Build history of the part. All positions in model axes, mm. Face numbers are marked on the shaded views. A direction names the side the tool comes from. Round coordinates to 2 decimals unless told otherwise and drop trailing zeros. Write each loop counter-clockwise with the first axis right and the second up, starting at its lowest first coordinate (ties: lowest second). Pieces come first, ordered by that corner, then holes. Notation, with made-up numbers: M 41,37.25 L 80,37.25 A16 cw 80,51.25 Z; hole C -13.75,66 d2. An arc over 180 degrees is marked long. Write item = value, one per line.
from build123d import *

# Parameters (mm, degrees)
SKETCH2_W                 = 39
SKETCH2_H                 = 29
BOSS_EXTRUDE1_DEPTH       = 14.5
SKETCH4_R                 = 14
BOSS_EXTRUDE2_DEPTH       = 6.5
SKETCH5_R                 = 21
BOSS_EXTRUDE3_DEPTH       = 40
SKETCH6_R                 = 27
BOSS_EXTRUDE4_DEPTH       = 15.5
M3X0_5_TAPPED_HOLE1_D     = 2.5
M3X0_5_TAPPED_HOLE1_DEPTH = 5
M3X0_5_TAPPED_HOLE1_TIP   = 0.751075774


with BuildPart() as part:
    # Sketch2 → Boss-Extrude1 (new, symmetric)
    with BuildSketch(Plane(origin=(0, 0, 0), x_dir=(1, 0, 0), z_dir=(0, 1, 0))):
        Rectangle(SKETCH2_W, SKETCH2_H)
    extrude(amount=BOSS_EXTRUDE1_DEPTH, both=True)

    # Sketch4 → Boss-Extrude2 (add)
    with BuildSketch(Plane(origin=(19.5, 0, 0), x_dir=(0, 0, -1), z_dir=(1, 0, 0))):
        with Locations(Location((0, 0, 0), (0, 0, 180))):
            Circle(SKETCH4_R)
    extrude(amount=BOSS_EXTRUDE2_DEPTH)

    # Sketch5 → Boss-Extrude3 (add)
    with BuildSketch(Plane(origin=(26, 0, 0), x_dir=(0, 0, -1), z_dir=(1, 0, 0))):
        Circle(SKETCH5_R)
    extrude(amount=BOSS_EXTRUDE3_DEPTH)

    # Sketch6 → Boss-Extrude4 (add)
    with BuildSketch(Plane(origin=(66, 0, 0), x_dir=(0, 0, -1), z_dir=(1, 0, 0))):
        Circle(SKETCH6_R)
    extrude(amount=BOSS_EXTRUDE4_DEPTH)

    # M3x0.5 Tapped Hole1
    with Locations(Plane(origin=(0, -14.5, 0), x_dir=(-1, 0, 0), z_dir=(0, -1, 0))):
        with Locations((-16.5, 11.5), (16.5, 11.5), (16.5, -11.5), (-16.5, -11.5)):
            Hole(M3X0_5_TAPPED_HOLE1_D / 2, depth=M3X0_5_TAPPED_HOLE1_DEPTH)
            with Locations((0, 0, -(M3X0_5_TAPPED_HOLE1_DEPTH + M3X0_5_TAPPED_HOLE1_TIP / 2))):  # 118° drill point
                Cone(0, M3X0_5_TAPPED_HOLE1_D / 2, M3X0_5_TAPPED_HOLE1_TIP, mode=Mode.SUBTRACT)

    # Sketch12 → Revolve1 (revolve)
    with BuildSketch(Plane.XY, mode=Mode.PRIVATE) as revolve1_sk:
        Polygon((61.5, 0), (141.5, 67.127970494), (141.5, 0), align=None)
    revolve(revolve1_sk.sketch.rotate(Axis((61.5, 0, 0), (1, 0, 0)), 270), axis=Axis((61.5, 0, 0), (1, 0, 0)))


solid = part.part
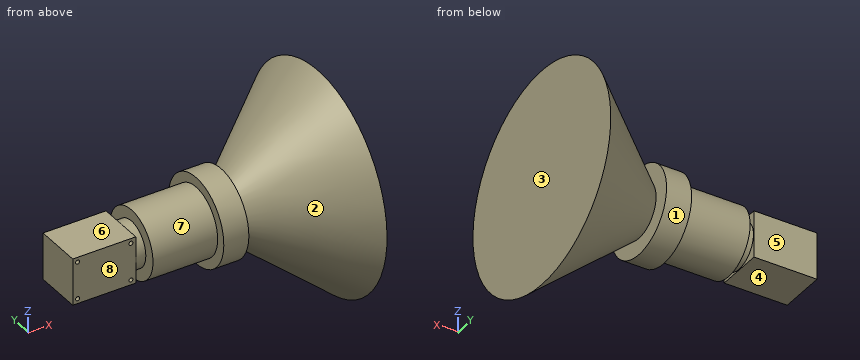
1. Probe probe 1 along Z at (x, y) = (16.5, -12.05); probe 2 along X at (y, z) = (-13, -11); probe 3 along Z at (x, y) = (16, -11). List the from-to ranges inside material, lowest first.
Responses:
probe_1 = -14.5 to -12.75, -10.25 to 10.25, 12.75 to 14.5
probe_2 = -19.5 to -17.65, -15.35 to 15.35, 17.65 to 19.5, 26 to 81.5, 81.79 to 141.5
probe_3 = -14.5 to -12.65, -10.35 to 10.35, 12.65 to 14.5
2. Band-saw the part on D-D (x = 112.5). List the corners of the cut face in (y, z), plus the area to 3 significant figures.
Responses:
outline = C 0,0 d85.59
area = 5,750 mm²
3. Tool access for the marked faces 4, 5, 6, 7 and 8: list every direction of +Z, -Z, +X, -X, +Y, -Y with a clear straight run to the whole face (end or side of a thin tool).
Responses:
face_4 = -Z, -X, +Y, -Y
face_5 = +Z, -Z, -X, +Y
face_6 = +Z, -X, +Y, -Y
face_7 = -X
face_8 = +Z, -Z, -X, -Y
4. Band-saw the part on A-A (z = 0). List the corners of the cut face in (x, y).
Responses:
outline = M -19.5,-14.5 L 19.5,-14.5 L 19.5,-14 L 26,-14 L 26,-21 L 66,-21 L 66,-27 L 81.5,-27 L 81.5,-16.78 L 141.5,-67.13 L 141.5,67.13 L 81.5,16.78 L 81.5,27 L 66,27 L 66,21 L 26,21 L 26,14 L 19.5,14 L 19.5,14.5 L -19.5,14.5 Z
5. Band-saw the part on C-C (x = 46). List the corners of the cut face in (y, z), plus the area to 3 significant figures.
Responses:
outline = C 0,0 d42
area = 1,390 mm²
6. Flat gauge pins, fed straight in: pin 1 (10 mm diameter, centred on x = 113, y = -34, fed in from -Z); pin 2 (10 mm diameter, centred on x = 13, z = 10, fed in from +Y); pin 3 (3 mm diameter, centred on x = -16.5, z = -11.5, fed in from -Y). Where does each tip first touch, or does it go through?
Responses:
pin_1 = -34.76
pin_2 = 14.5
pin_3 = -14.5
7. Mould opens along X. For the marked faces 1, 2 and 3 say: pulls with the +X half, pulls with the -X half, needs draft (parallel to the pull), parting line crosses it, or undercut.
Responses:
face_1 = needs draft
face_2 = undercut
face_3 = pulls with the +X half
